For this review, take the finished solid that the model builds, in its own axes (mm). A direction names the side the tool comes from. Round coordinates to 2 decimals unless told otherwise and drop trailing zeros. Order: outer loops, then holes, each group sorted by start corner. A loop starts at its lowest first (then second) coordinate and runs counter-clockwise, first axis right, second up. Notation, with made-up numbers: (-0.75, 4) -> (22.25, 4) arc R25 ccw to (22.25, 19) -> close; hole circle Ø11 at (31, 12.5). An arc over 180 degrees is marked (long way). Put each result on its own line as item: value. Start each with the question number.
```python
from build123d import *

# Parameters (mm, degrees)
EXTRUDE1_DEPTH          = 2.794
HOLE1_D                 = 1.459992
HOLE1_CBORE_D           = 1.89992
HOLE1_CBORE_DEPTH       = 0.89408
EXTRUDE2_DEPTH          = 2.794
HOLE_PATTERN_COUNT      = 32
HOLE_PATTERN_PITCH      = 2.54
HOLE_PATTERN_COUNT_DIR2 = 2
HOLE_PATTERN_PITCH_DIR2 = 2.54
SLOT_PATTERN_COUNT      = 31
SLOT_PATTERN_PITCH      = 2.54


with BuildPart() as part:
    # Sketch1 → Extrude1 (new body)
    with BuildSketch(Plane(origin=(0, 0, 0), x_dir=(1, 0, 0), z_dir=(0, 1, 0))):
        Polygon((20.014373708, 0.40005), (19.854353708, 0.40005), (19.708747416, 0), (0, 0), (-0.145606292, 0.40005), (-0.305626292, 0.40005), (-0.305626292, 4.67995), (-0.145606292, 4.67995), (0, 5.08), (19.708747416, 5.08), (19.854353708, 4.67995), (20.014373708, 4.67995), align=None)
    extrude(amount=-EXTRUDE1_DEPTH)

    # Hole1 (through all)
    with Locations(Plane(origin=(0.964373708, 0, -1.27), x_dir=(0, 0, 1), z_dir=(0, 1, 0))):
        with Locations((0, 0)):
            hole1 = CounterBoreHole(HOLE1_D / 2, HOLE1_CBORE_D / 2, HOLE1_CBORE_DEPTH)

    # Sketch4 → Extrude2 (cut)
    with BuildSketch(Plane(origin=(0, 0, 0), x_dir=(1, 0, 0), z_dir=(0, 1, 0))):
        Polygon((1.928772816, 0), (2.5399746, 0), (2.394368308, 0.40005), (2.074379108, 0.40005), align=None)
        Polygon((2.074379108, 4.67995), (2.394368308, 4.67995), (2.5399746, 5.08), (1.928772816, 5.08), align=None)
    extrude2 = extrude(amount=-EXTRUDE2_DEPTH, mode=Mode.SUBTRACT)

    # Hole Pattern: Hole1 32 × 2
    with Locations(*[(i * HOLE_PATTERN_PITCH, 0, -j * HOLE_PATTERN_PITCH_DIR2) for i in range(HOLE_PATTERN_COUNT) for j in range(HOLE_PATTERN_COUNT_DIR2) if (i, j) != (0, 0)]):
        add(hole1, mode=Mode.SUBTRACT)

    # Slot Pattern: Extrude2 ×31
    with Locations(*[(i * SLOT_PATTERN_PITCH, 0, 0) for i in range(1, SLOT_PATTERN_COUNT)]):
        add(extrude2, mode=Mode.SUBTRACT)


solid = part.part
```
Item 1: For L1, parallel to Z at x = 9, y = -2.4; L2, parallel to Z at x = 3, y = -2.1; L3, parallel to Y at x = 14.5, z = -3.7, list the stretches that pass through material, from the lowest coordinate up.
Item 2: Insertion check: pin 1 Ø0.9 at (x, z) = (14, -1.5) entering from +Y. The pin has a flat end and moves straight along its axis. Give the tip position at first contact, or say it passes through.
Item 3: Mouldability with a two-part tool opening along Z and no side actions: class faces 1 (the face through (14, -1, -5.08)), 2 (the face through (6.845, -0.441, -3.299)), 3 (the face through (14, -1, 0)) as +Z half, -Z half, draft (parallel to the pull), parting line (faces both ways), or undercut.
Item 4: Consider section D-D, the plane x = 18.25. Write out the cut boundary in (y, z).
Item 5: Consider section B-B, the plane z = -1.27. Count the separate pieces of the cut face and the enclosed holes in it, plus the area to 3 significant figures.
Item 6: Tool access review of faces 4 (the face through (6, -1, -5.08)), 5 (the face through (6.986, -0.441, -1.394)): name each direction out of +Z, -Z, +X, -X, +Y, -Y from which nothing blocks a thin tool from reaching the whole face with its end or side.
Item 7: Consider section A-A, the plane x = 6.5. Write out the cut boundary in (y, z), plus the area to 3 significant figures.
Evaluation:
1. L1: z = -5.08 to -4.41, -3.21 to -1.87, -0.67 to 0
1. L2: z = -5.08 to -4.34, -3.28 to -1.8, -0.74 to 0
1. L3: y = -2.79 to -0.89
2. pin 1: stops at y = -0.89
3. face 1: -Z half
3. face 2: undercut
3. face 3: +Z half
4. outline: (-2.79, -5.08) -> (0, -5.08) -> (0, -4.62) -> (-0.89, -4.62) -> (-0.89, -4.35) -> (-2.79, -4.35) -> close; (-2.79, -3.27) -> (-0.89, -3.27) -> (-0.89, -3) -> (0, -3) -> (0, -2.08) -> (-0.89, -2.08) -> (-0.89, -1.81) -> (-2.79, -1.81) -> close; (-2.79, -0.73) -> (-0.89, -0.73) -> (-0.89, -0.46) -> (0, -0.46) -> (0, 0) -> (-2.79, 0) -> close
5. separate pieces: 9
5. enclosed holes: 0
5. area: 21.0 mm^2
6. face 4: -Z, +X, -X, +Y, -Y
6. face 5: +Y
7. outline: (-2.79, -5.08) -> (0, -5.08) -> (0, -4.64) -> (-0.89, -4.64) -> (-0.89, -4.38) -> (-2.79, -4.38) -> close; (-2.79, -3.24) -> (-0.89, -3.24) -> (-0.89, -2.98) -> (0, -2.98) -> (0, -2.1) -> (-0.89, -2.1) -> (-0.89, -1.84) -> (-2.79, -1.84) -> close; (-2.79, -0.7) -> (-0.89, -0.7) -> (-0.89, -0.44) -> (0, -0.44) -> (0, 0) -> (-2.79, 0) -> close
7. area: 6.88 mm^2
